Build history of the part. All positions in model axes, mm. A direction names the side the tool comes from. Give positions to 0.01 mm unless a question says otherwise; leave off trailing zeros. Write each loop counter-clockwise with the first axis right and the second up, starting at its lowest first coordinate (ties: lowest second). Pieces come first, ordered by that corner, then holes. Notation, with made-up numbers: M -39,36.5 L -22,36.5 A22 ccw -22,75.5 Z; hole C -8.5,84.5 d1. An arc over 180 degrees is marked long. Return JSON: item names as keys, results as strings. Group by question number.
Q1. Wall check: probe 1 along X at (y, z) = (51.5, 23.5); probe 2 along X at (y, z) = (27.5, 27); probe 3 along X at (y, z) = (18.5, 6.5). Give the ranges that are in metal, low to high.
Q2. Band-saw the part on C-C, the plane z = 14. Count the separate pieces of the cut face and the enclosed holes in it, then the cut area to 3 significant figures.
Q3. Pull direction X, two halves, no side cores. Call faces 5 (the cylindrical face through (-9.958, -19.676, 7.998)), 6 (the flat face through (5, 35, 0)), 7 (the cylindrical face through (11.43, -39, 18.78)): +X half, -X half, draft (parallel to the pull), parting line (faces both ways), or undercut.
Q4. Band-saw the part on B-B, the plane x = -32. Give the cut face in (y, z), then the cut area to 3 significant figures.
Q5. Band-saw the part on D-D, the plane x = 23.5. Give the cut face in (y, z), then the cut area to 3 significant figures.
Q6. Band-saw the part on A-A, the plane y = -2.5. Give the cut face in (x, z), then the cut area to 3 significant figures.
Q7. Flat gauge pins, fed straight in: pin 1 Ø9.5 at (y, z) = (-1, 23.5) entering from -X; pin 2 Ø4 at (x, z) = (21.5, 6) entering from -Y; pin 3 Ø3.5 at (x, y) = (32, -36.5) entering from +Z; pin 4 Ø2.5 at (x, y) = (-32, -36.5) entering from -Z. Where does each tip first touch, or does it go through?
Q8. Tool access for faces 1 (the flat face through (10, -47, 19)), 2 (the flat face through (8, 48, 17)), 3 (the flat face through (0, -57.5, 19)), 4 (the flat face through (27, 11, 16)): list every direction of +Z, -Z, +X, -X, +Y, -Y with a clear straight run to the whole face (end or side of a thin tool).
from build123d import *

# Parameters (mm, degrees)
SKETCH1_W           = 70
SKETCH1_H           = 119
BOSS_EXTRUDE1_DEPTH = 35
SKETCH2_R           = 8
CUT_EXTRUDE1_DEPTH  = 8
SKETCH3_R           = 8
CUT_EXTRUDE2_DEPTH  = 8
SKETCH4_W           = 14
SKETCH4_H           = 89
CUT_EXTRUDE3_DEPTH  = 32
CUT_EXTRUDE4_REACH  = 82.804
CUT_EXTRUDE5_REACH  = 82.804
SKETCH7_W           = 23
SKETCH7_H           = 20
SKETCH7_W_2         = 16
CUT_EXTRUDE7_DEPTH  = 78.396705356
CUT_EXTRUDE8_DEPTH  = 5
SKETCH12_W          = 18
SKETCH12_H          = 32
CUT_EXTRUDE9_DEPTH  = 2
SKETCH13_W          = 24
SKETCH13_H          = 32
CUT_EXTRUDE10_DEPTH = 2
SKETCH14_W          = 23
SKETCH14_H          = 32
CUT_EXTRUDE11_DEPTH = 2
SKETCH15_W          = 32
SKETCH15_H          = 20
CUT_EXTRUDE12_DEPTH = 2
SKETCH16_W          = 32
SKETCH16_H          = 20
CUT_EXTRUDE13_DEPTH = 2
SKETCH17_W          = 65
SKETCH17_H          = 32
CUT_EXTRUDE15_DEPTH = 2
SKETCH18_W          = 16
SKETCH18_H          = 32
CUT_EXTRUDE16_DEPTH = 2
CUT_EXTRUDE17_DEPTH = 5
SKETCH21_R          = 1.5
CUT_EXTRUDE18_DEPTH = 10
FILLET1_R           = 5
FILLET2_R           = 5


with BuildPart() as part:
    # Sketch1 → Boss-Extrude1 (new body)
    with BuildSketch(Plane.XY):
        Rectangle(SKETCH1_W, SKETCH1_H)
    extrude(amount=BOSS_EXTRUDE1_DEPTH)

    # Sketch2 → Cut-Extrude1 (cut)
    with BuildSketch(Plane(origin=(35, 0, 0), x_dir=(0, 0, -1), z_dir=(1, 0, 0))):
        with Locations((0, -19.5)):
            Circle(SKETCH2_R)
    extrude(amount=-CUT_EXTRUDE1_DEPTH, mode=Mode.SUBTRACT)

    # Sketch3 → Cut-Extrude2 (cut)
    with BuildSketch(Plane.ZY.offset(35)):
        with Locations((0, 19.5)):
            Circle(SKETCH3_R)
    extrude(amount=-CUT_EXTRUDE2_DEPTH, mode=Mode.SUBTRACT)

    # Sketch4 → Cut-Extrude3 (cut)
    with BuildSketch(Plane(origin=(0, 0, 0), x_dir=(-1, 0, 0), z_dir=(0, 0, -1))):
        Polygon((-13, -34.5), (-13, 54.5), (-27, 54.5), (-27, -11.5), (-27, -27.5), (-27, -34.5), align=None)
        with Locations((0, -10)):
            Rectangle(SKETCH4_W, SKETCH4_H)
        Polygon((27, 54.5), (13, 54.5), (13, -34.5), (27, -34.5), (27, 11.5), (27, 27.5), align=None)
    extrude(amount=-CUT_EXTRUDE3_DEPTH, mode=Mode.SUBTRACT)

    # Sketch5 → Cut-Extrude4 (cut, up to next)
    with BuildSketch(Plane.ZY.offset(-7), mode=Mode.PRIVATE) as cut_extrude4_sk1:
        with BuildLine():
            Line((0, 27.5), (0, 11.5))
            ThreePointArc((0, 11.5), (8, 19.5), (0, 27.5))
        make_face()
    cut_extrude4_tool1 = extrude(cut_extrude4_sk1.sketch, amount=-CUT_EXTRUDE4_REACH, mode=Mode.PRIVATE) & part.part
    add(cut_extrude4_tool1.solids().sort_by_distance((7, 19.5, 3.395305))[0], mode=Mode.SUBTRACT)

    # Sketch6 → Cut-Extrude5 (cut, up to next)
    with BuildSketch(Plane(origin=(-7, 0, 0), x_dir=(0, 0, -1), z_dir=(1, 0, 0)), mode=Mode.PRIVATE) as cut_extrude5_sk1:
        with BuildLine():
            Line((0, -11.5), (0, -27.5))
            ThreePointArc((0, -27.5), (-8, -19.5), (0, -11.5))
        make_face()
    cut_extrude5_tool1 = extrude(cut_extrude5_sk1.sketch, amount=-CUT_EXTRUDE5_REACH, mode=Mode.PRIVATE) & part.part
    add(cut_extrude5_tool1.solids().sort_by_distance((-7, -19.5, 3.395305))[0], mode=Mode.SUBTRACT)

    # Sketch7 → Cut-Extrude7 (cut, through all)
    with BuildSketch(Plane(origin=(0, 0, 0), x_dir=(-1, 0, 0), z_dir=(0, 0, -1))):
        with Locations((23.5, -49.5)):
            Rectangle(SKETCH7_W, SKETCH7_H)
        with Locations((0, 49.5)):
            Rectangle(SKETCH7_W_2, SKETCH7_H)
        with Locations((-23.5, -49.5)):
            Rectangle(SKETCH7_W, SKETCH7_H)
    extrude(amount=-CUT_EXTRUDE7_DEPTH, mode=Mode.SUBTRACT)

    # Sketch11 → Cut-Extrude8 (cut)
    with BuildSketch(Plane(origin=(35, 0, 0), x_dir=(0, 0, -1), z_dir=(1, 0, 0))):
        with BuildLine():
            Line((-3, 59.5), (-35, 59.5))
            Line((-35, 59.5), (-35, -39.5))
            Line((-35, -39.5), (-3, -39.5))
            Line((-3, -39.5), (-3, -30.083005244))
            ThreePointArc((-3, -30.083005244), (-11, -19.5), (-3, -8.916994756))
            Line((-3, -8.916994756), (-3, 59.5))
        make_face()
    extrude(amount=-CUT_EXTRUDE8_DEPTH, mode=Mode.SUBTRACT)

    # Sketch12 → Cut-Extrude9 (cut)
    with BuildSketch(Plane.XZ.offset(39.5)):
        with Locations((21, 19)):
            Rectangle(SKETCH12_W, SKETCH12_H)
    extrude(amount=-CUT_EXTRUDE9_DEPTH, mode=Mode.SUBTRACT)

    # Sketch13 → Cut-Extrude10 (cut)
    with BuildSketch(Plane.XZ.offset(59.5)):
        with Locations((0, 19)):
            Rectangle(SKETCH13_W, SKETCH13_H)
    extrude(amount=-CUT_EXTRUDE10_DEPTH, mode=Mode.SUBTRACT)

    # Sketch14 → Cut-Extrude11 (cut)
    with BuildSketch(Plane.XZ.offset(39.5)):
        with Locations((-23.5, 19)):
            Rectangle(SKETCH14_W, SKETCH14_H)
    extrude(amount=-CUT_EXTRUDE11_DEPTH, mode=Mode.SUBTRACT)

    # Sketch15 → Cut-Extrude12 (cut)
    with BuildSketch(Plane.ZY.offset(12)):
        with Locations((19, -47.5)):
            Rectangle(SKETCH15_W, SKETCH15_H)
    extrude(amount=-CUT_EXTRUDE12_DEPTH, mode=Mode.SUBTRACT)

    # Sketch16 → Cut-Extrude13 (cut)
    with BuildSketch(Plane(origin=(12, 0, 0), x_dir=(0, 0, -1), z_dir=(1, 0, 0))):
        with Locations((-19, -47.5)):
            Rectangle(SKETCH16_W, SKETCH16_H)
    extrude(amount=-CUT_EXTRUDE13_DEPTH, mode=Mode.SUBTRACT)

    # Sketch17 → Cut-Extrude15 (cut)
    with BuildSketch(Plane(origin=(0, 59.5, 0), x_dir=(1, 0, 0), z_dir=(0, 1, 0))):
        with Locations((-2.5, -19)):
            Rectangle(SKETCH17_W, SKETCH17_H)
    extrude(amount=-CUT_EXTRUDE15_DEPTH, mode=Mode.SUBTRACT)

    # Sketch18 → Cut-Extrude16 (cut)
    with BuildSketch(Plane(origin=(0, 39.5, 0), x_dir=(1, 0, 0), z_dir=(0, 1, 0))):
        with Locations((0, -19)):
            Rectangle(SKETCH18_W, SKETCH18_H)
    extrude(amount=-CUT_EXTRUDE16_DEPTH, mode=Mode.SUBTRACT)

    # Sketch19 → Cut-Extrude17 (cut)
    with BuildSketch(Plane.ZY.offset(35)):
        with BuildLine():
            Line((3, 57.5), (35, 57.5))
            Line((35, 57.5), (35, -37.5))
            Line((35, -37.5), (3, -37.5))
            Line((3, -37.5), (3, 8.916994756))
            ThreePointArc((3, 8.916994756), (11, 19.5), (3, 30.083005244))
            Line((3, 30.083005244), (3, 57.5))
        make_face()
    extrude(amount=-CUT_EXTRUDE17_DEPTH, mode=Mode.SUBTRACT)

    # Sketch21 → Cut-Extrude18 (cut)
    with BuildSketch(Plane(origin=(0, 0, 0), x_dir=(-1, 0, 0), z_dir=(0, 0, -1))):
        with Locations((-32, 56.5)):
            Circle(SKETCH21_R)
        with Locations((32, 56.5)):
            Circle(SKETCH21_R)
        with Locations((-32, -36.5)):
            Circle(SKETCH21_R)
        with Locations((32, -36.5)):
            Circle(SKETCH21_R)
    extrude(amount=-CUT_EXTRUDE18_DEPTH, mode=Mode.SUBTRACT)

    # Fillet1
    fillet1_edges = [part.edges().sort_by_distance(p)[0] for p in [
        (-30, 57.5, 19),
        (-8, 57.5, 19),
        (-8, 37.5, 19),
        (8, 37.5, 19),
        (8, 57.5, 19),
        (30, 57.5, 19),
        (30, -37.5, 19),
        (10, -37.5, 19),
        (10, -57.5, 19),
        (-10, -37.5, 19),
        (-30, -37.5, 19),
        (-10, -57.5, 19),
    ]]
    fillet(fillet1_edges, radius=FILLET1_R)

    # Fillet2
    fillet2_edges = [part.edges().sort_by_distance(p)[0] for p in [
        (35, -39.5, 1.5),
        (35, 59.5, 1.5),
        (12, -39.5, 1.5),
        (12, -59.5, 1.5),
        (-12, -59.5, 1.5),
        (-12, -39.5, 1.5),
        (-35, -39.5, 1.5),
        (-8, 59.5, 1.5),
        (8, 59.5, 1.5),
        (-35, 59.5, 1.5),
    ]]
    fillet(fillet2_edges, radius=FILLET2_R)


solid = part.part
From the geometry:
{
 "1": {"probe 1": "x = -30 to -27, -13 to -8, 8 to 13, 27 to 30", "probe 2": "x = -30 to -27, -13 to -7, 7 to 13, 27 to 30", "probe 3": "x = -13 to -7, 27 to 30"},
 "2": {"separate pieces": "1", "enclosed holes": "3", "area": "2,020 mm^2"},
 "3": {"face 5": "undercut", "face 6": "draft", "face 7": "+X half"},
 "4": {"outline": "M -39.08,0 L -38,0 L -38,3 L -39.08,3 Z; M -35,0 L 11.5,0 A8 cw 27.5,0 L 55,0 L 55,3 L 30.08,3 A11 ccw 8.92,3 L -35,3 Z; M 58,0 L 59.08,0 L 59.08,3 L 58,3 Z", "area": "301 mm^2"},
 "5": {"outline": "M -39.5,0 L -34.5,0 L -34.5,32 L 54.5,32 L 54.5,0 L 59.5,0 L 59.5,3 L 57.5,3 L 57.5,35 L -37.5,35 L -37.5,3 L -39.5,3 Z", "area": "489 mm^2"},
 "6": {"outline": "M -35,0 L -27,0 L -27,32 L -13,32 L -13,0 L -7,0 L -7,32 L 7,32 L 7,0 L 13,0 L 13,32 L 27,32 L 27,0 L 35,0 L 35,3 L 30,3 L 30,35 L -30,35 L -30,3 L -35,3 Z", "area": "786 mm^2"},
 "7": {"pin 1": "stops at x = -30", "pin 2": "stops at y = -37.5", "pin 3": "stops at z = 3", "pin 4": "passes through"},
 "8": {"face 1": "+Z, +X, -Y", "face 2": "+Z, -Z, +Y", "face 3": "+Z, +X, -X, -Y", "face 4": "-Z"}
}
